from build123d import *

# Parameters (mm, degrees)
SKETCH6_R              = 1.6
SKETCH6_R_2            = 2.575
SKETCH6_W              = 5
SKETCH6_H              = 5
SKETCH6_H_2            = 5.1
SKETCH6_R_3            = 2.05
SKETCH6_R_4            = 4.707512696
BOSS_EXTRUDE4_DEPTH    = 2
SKETCH7_R              = 1.6
SKETCH7_R_2            = 2.575
BOSS_EXTRUDE5_DEPTH    = 5
SKETCH8_R              = 1.6
MIDSECTION_HOLES_DEPTH = 8
SKETCH12_R             = 4.575
BOSS_EXTRUDE6_DEPTH    = 6
SKETCH13_R             = 2.575
CUT_EXTRUDE4_DEPTH     = 4
FILLET1_R              = 0.5


with BuildPart() as part:
    # Sketch6 → Boss-Extrude4 (new body)
    with BuildSketch(Plane.XY):
        with BuildLine():
            Line((25, 17.15), (-110, 17.15))
            ThreePointArc((-110, 17.15), (-127.15, 0), (-110, -17.15))
            Line((-110, -17.15), (25, -17.15))
            ThreePointArc((25, -17.15), (42.15, 0), (25, 17.15))
        make_face()
        with Locations((-31, -13.6)):
            Circle(SKETCH6_R, mode=Mode.SUBTRACT)
        with Locations((-11, -13.6)):
            Circle(SKETCH6_R, mode=Mode.SUBTRACT)
        with Locations((-110, 0)):
            Circle(SKETCH6_R_2, mode=Mode.SUBTRACT)
        with Locations((13.6, 0)):
            Rectangle(SKETCH6_W, SKETCH6_H, mode=Mode.SUBTRACT)
        with Locations((25, 0)):
            Circle(SKETCH6_R_2, mode=Mode.SUBTRACT)
        with Locations((-31, 13.6)):
            Circle(SKETCH6_R, mode=Mode.SUBTRACT)
        with Locations((-11, 13.6)):
            Circle(SKETCH6_R, mode=Mode.SUBTRACT)
        with Locations((-31, 0)):
            Rectangle(SKETCH6_W, SKETCH6_H_2, mode=Mode.SUBTRACT)
        with Locations((-11, 0)):
            Circle(SKETCH6_R_3, mode=Mode.SUBTRACT)
        Circle(SKETCH6_R_4, mode=Mode.SUBTRACT)
        with Locations((-20, 8.75)):
            Circle(SKETCH6_R, mode=Mode.SUBTRACT)
        with Locations((-20, -8.75)):
            Circle(SKETCH6_R, mode=Mode.SUBTRACT)
    extrude(amount=BOSS_EXTRUDE4_DEPTH)

    # Sketch7 → Boss-Extrude5 (add)
    with BuildSketch(Plane.XY.offset(2)):
        with BuildLine():
            Line((25, 17.15), (-110, 17.15))
            ThreePointArc((-110, 17.15), (-127.15, 0), (-110, -17.15))
            Line((-110, -17.15), (25, -17.15))
            ThreePointArc((25, -17.15), (42.15, 0), (25, 17.15))
        make_face()
        with Locations((-31, -13.6)):
            Circle(SKETCH7_R, mode=Mode.SUBTRACT)
        with Locations((-11, -13.6)):
            Circle(SKETCH7_R, mode=Mode.SUBTRACT)
        with Locations((-110, 0)):
            Circle(SKETCH7_R_2, mode=Mode.SUBTRACT)
        Polygon((-51.9, -11.15), (-51.9, 11.15), (11.1, 11.15), (11.1, 2.5), (16.1, 2.5), (16.1, -2.5), (11.1, -2.5), (11.1, -11.15), align=None, mode=Mode.SUBTRACT)
        with Locations((25, 0)):
            Circle(SKETCH7_R_2, mode=Mode.SUBTRACT)
        with Locations((-31, 13.6)):
            Circle(SKETCH7_R, mode=Mode.SUBTRACT)
        with Locations((-11, 13.6)):
            Circle(SKETCH7_R, mode=Mode.SUBTRACT)
    extrude(amount=BOSS_EXTRUDE5_DEPTH)

    # Sketch8 → midsection_holes (cut, through all)
    with BuildSketch(Plane.XY.offset(7)):
        with Locations((-75, 3.75)):
            Circle(SKETCH8_R)
        with Locations((-67.5, -3.75)):
            Circle(SKETCH8_R)
    extrude(amount=-MIDSECTION_HOLES_DEPTH, mode=Mode.SUBTRACT)

    # Sketch12 → Boss-Extrude6 (add)
    with BuildSketch(Plane.XY.offset(7)):
        with Locations((-110, 0)):
            Circle(SKETCH12_R)
        with Locations((25, 0)):
            Circle(SKETCH12_R)
    extrude(amount=BOSS_EXTRUDE6_DEPTH)

    # Sketch13 → Cut-Extrude4 (cut)
    with BuildSketch(Plane(origin=(0, 0, 7), x_dir=(-1, 0, 0), z_dir=(0, 0, -1))):
        with Locations((-25, 0)):
            Circle(SKETCH13_R)
        with Locations((110, 0)):
            Circle(SKETCH13_R)
    extrude(amount=-CUT_EXTRUDE4_DEPTH, mode=Mode.SUBTRACT)

    # Fillet1
    fillet1_edges = [part.edges().sort_by_distance(p)[0] for p in [
        (-114.575, 0, 13),
        (20.425, 0, 13),
        (-127.15, 0, 7),
        (-42.5, -17.15, 7),
        (42.15, 0, 7),
        (-42.5, 17.15, 7),
    ]]
    fillet(fillet1_edges, radius=FILLET1_R)


solid = part.part
Geometry: final body of the model. Coordinates: model frame, mm. A direction names the side the tool comes from. Give positions to 0.01 mm unless a question says otherwise; leave off trailing zeros. Write each loop counter-clockwise with the first axis right and the second up, starting at its lowest first coordinate (ties: lowest second). Pieces come first, ordered by that corner, then holes. Notation, with made-up numbers: (-28.5, -37) -> (11.5, -37) arc R29 ccw to (11.5, -7) -> close; hole circle Ø6 at (-20.5, 77.5). An arc over 180 degrees is marked (long way). Answer as a JSON object with one key per item and string values.
1. Mould query, pull axis Y, two halves, no side actions, for faces 1 (the flat face through (25, 0, 13)), 2 (the flat face through (-42, 17.15, 3)), 3 (the flat face through (14, 2.5, 3)), 4 (the cylindrical face through (42.146, -0.377, 3.204)). Classes: pulls with the +Y half, pulls with the -Y half, needs draft (parallel to the pull), parting line crosses it, or undercut.
Ans:
{"face 1": "needs draft", "face 2": "pulls with the +Y half", "face 3": "undercut", "face 4": "parting line crosses it"}
2. Cut plane C-C on x = -67.5. Output: boundary loops of the cut face in (y, z), and give its area (3 significant figures).
Ans:
{"outline": "(-17.15, 0) -> (-5.35, 0) -> (-5.35, 7) -> (-16.65, 7) arc R0.5 ccw to (-17.15, 6.5) -> close; (-2.15, 0) -> (17.15, 0) -> (17.15, 6.5) arc R0.5 ccw to (16.65, 7) -> (-2.15, 7) -> close", "area": "218 mm^2"}
3. Ray query, probe 1 along X at (y, z) = (0, 4) (3 decimals); probe 2 along Y at (x, z) = (-11, 3); probe 3 along Y at (x, z) = (25, 8.75) (3 decimals). Return the intervals inside material, ascending. Write a range as from..to.
Ans:
{"probe 1": "x = -127.15..-112.575, -107.425..-51.9, 16.1..22.425, 27.575..42.15", "probe 2": "y = -17.15..-15.2, -12..-11.15, 11.15..12, 15.2..17.15", "probe 3": "y = -4.575..-2.575, 2.575..4.575"}
4. Access query for faces 5 (the flat face through (16.1, 0, 3)), 6 (the flat face through (-43, -17.15, 3)), 7 (the flat face through (-51.9, 0, 4)). Directions: +Z, -Z, +X, -X, +Y, -Y. A direction counts if a zero-diameter tool reaches every point of the face in a straight line with its end or side. Return the directions, or none.
Ans:
{"face 5": "+Z, -Z", "face 6": "+Z, -Z, +X, -X, -Y", "face 7": "+Z"}
5. Contact query for flat-ended pins moving along their axis: pin 1 (3 mm diameter, centred on x = 25, y = 0, fed in from -Z); pin 2 (4 mm diameter, centred on x = 23, y = -11.5, fed in from +Z); pin 3 (1.9 mm diameter, centred on x = -11, y = -13.6, fed in from -Z); pin 4 (5 mm diameter, centred on y = -11.5, z = 7.5, fed in from -X). Output: stop coordinate, or through.
Ans:
{"pin 1": "stops at z = 11", "pin 2": "stops at z = 7", "pin 3": "passes through", "pin 4": "stops at x = -124.48"}
6. Cut plane A-A on x = -20. Output: boundary loops of the cut face in (y, z), and give its area (3 significant figures).
Ans:
{"outline": "(-17.15, 0) -> (-10.35, 0) -> (-10.35, 2) -> (-11.15, 2) -> (-11.15, 7) -> (-16.65, 7) arc R0.5 ccw to (-17.15, 6.5) -> close; (-7.15, 0) -> (7.15, 0) -> (7.15, 2) -> (-7.15, 2) -> close; (10.35, 0) -> (17.15, 0) -> (17.15, 6.5) arc R0.5 ccw to (16.65, 7) -> (11.15, 7) -> (11.15, 2) -> (10.35, 2) -> close", "area": "116 mm^2"}
7. Cut plane B-B on z = 4.5. Count the separate pieces of the cut face and the enclosed holes in it, and give its area (3 significant figures).
Ans:
{"separate pieces": "1", "enclosed holes": "9", "area": "4,030 mm^2"}
